```python
from build123d import *

# Parameters (mm, degrees)
SKETCH1_W           = 600
SKETCH1_H           = 540
BOSS_EXTRUDE1_DEPTH = 15
SKETCH2_W           = 175
SKETCH2_H           = 75.5
CUT_EXTRUDE1_DEPTH  = 404.887360535
SKETCH4_W           = 17
SKETCH4_H           = 32
CUT_EXTRUDE3_DEPTH  = 404.887360535
FILLET3_R           = 10
SKETCH5_W           = 40
SKETCH5_H           = 6
BOSS_EXTRUDE2_DEPTH = 15
SKETCH6_R           = 2.5
CUT_EXTRUDE4_DEPTH  = 404.887360535
BOSS_EXTRUDE3_DEPTH = 15
FILLET4_R           = 35
CUT_EXTRUDE5_DEPTH  = 15
FILLET5_R           = 7
SKETCH9_W           = 600
SKETCH9_H           = 5.5
CUT_EXTRUDE6_DEPTH  = 497.235831032
FILLET7_R           = 10
FILLET8_R           = 2
SKETCH10_W          = 90
SKETCH10_H          = 178
CUT_EXTRUDE7_DEPTH  = 15
FILLET9_R           = 5
SKETCH11_R          = 2.1
CUT_EXTRUDE8_DEPTH  = 15
SKETCH12_R          = 2
CUT_EXTRUDE9_DEPTH  = 497.235831032
SKETCH13_R          = 2
CUT_EXTRUDE10_DEPTH = 497.235831032


with BuildPart() as part:
    # Sketch1 → Boss-Extrude1 (new body)
    with BuildSketch(Plane.XY):
        Rectangle(SKETCH1_W, SKETCH1_H)
    extrude(amount=BOSS_EXTRUDE1_DEPTH)

    # Sketch2 → Cut-Extrude1 (cut, through all)
    with BuildSketch(Plane.XY.offset(15)):
        with Locations((-186, -232.25)):
            Rectangle(SKETCH2_W, SKETCH2_H)
        with Locations((186, -232.25)):
            Rectangle(SKETCH2_W, SKETCH2_H)
    extrude(amount=-CUT_EXTRUDE1_DEPTH, mode=Mode.SUBTRACT)

    # Sketch4 → Cut-Extrude3 (cut, through all)
    with BuildSketch(Plane.XY.offset(15)):
        with Locations((-259.5, 244.5)):
            Rectangle(SKETCH4_W, SKETCH4_H)
        with Locations((-112.5, 244.5)):
            Rectangle(SKETCH4_W, SKETCH4_H)
        with Locations((-259.5, -55.5)):
            Rectangle(SKETCH4_W, SKETCH4_H)
        with Locations((-112.5, -55.5)):
            Rectangle(SKETCH4_W, SKETCH4_H)
        with Locations((112.5, -55.5)):
            Rectangle(SKETCH4_W, SKETCH4_H)
        with Locations((259.5, -55.5)):
            Rectangle(SKETCH4_W, SKETCH4_H)
        with Locations((112.5, 244.5)):
            Rectangle(SKETCH4_W, SKETCH4_H)
        with Locations((259.5, 244.5)):
            Rectangle(SKETCH4_W, SKETCH4_H)
    extrude(amount=-CUT_EXTRUDE3_DEPTH, mode=Mode.SUBTRACT)

    # Fillet3
    fillet3_edges = [part.edges().sort_by_distance(p)[0] for p in [
        (-273.5, -194.5, 7.5),
        (-98.5, -194.5, 7.5),
        (98.5, -194.5, 7.5),
        (273.5, -194.5, 7.5),
    ]]
    fillet(fillet3_edges, radius=FILLET3_R)

    # Sketch5 → Boss-Extrude2 (add)
    with BuildSketch(Plane.XY.offset(15)):
        with Locations((-186, -197.5)):
            Rectangle(SKETCH5_W, SKETCH5_H)
        with Locations((186, -197.5)):
            Rectangle(SKETCH5_W, SKETCH5_H)
    extrude(amount=-BOSS_EXTRUDE2_DEPTH)

    # Sketch6 → Cut-Extrude4 (cut, through all)
    with BuildSketch(Plane.XY.offset(15)):
        with Locations((58.3, 117)):
            Circle(SKETCH6_R)
        with Locations((58.3, 103)):
            Circle(SKETCH6_R)
    extrude(amount=-CUT_EXTRUDE4_DEPTH, mode=Mode.SUBTRACT)

    # Sketch7 → Boss-Extrude3 (add)
    with BuildSketch(Plane.XY.offset(15)):
        Polygon((-300, 270), (300, 270), (175, 395), (-175, 395), align=None)
    extrude(amount=-BOSS_EXTRUDE3_DEPTH)

    # Fillet4
    fillet4_edges = [part.edges().sort_by_distance(p)[0] for p in [
        (-175, 395, 7.5),
        (175, 395, 7.5),
        (-300, 270, 7.5),
        (300, 270, 7.5),
    ]]
    fillet(fillet4_edges, radius=FILLET4_R)

    # Sketch8 → Cut-Extrude5 (cut)
    with BuildSketch(Plane.XY.offset(15)):
        Polygon((-230, 286.966991411), (-150, 286.966991411), (-150, 366.966991411), align=None)
        Polygon((150, 366.966991411), (230, 286.966991411), (150, 286.966991411), align=None)
    extrude(amount=-CUT_EXTRUDE5_DEPTH, mode=Mode.SUBTRACT)

    # Fillet5
    fillet5_edges = [part.edges().sort_by_distance(p)[0] for p in [
        (-230, 286.966991411, 7.5),
        (-150, 366.966991411, 7.5),
        (-150, 286.966991411, 7.5),
        (150, 286.966991411, 7.5),
        (150, 366.966991411, 7.5),
        (230, 286.966991411, 7.5),
    ]]
    fillet(fillet5_edges, radius=FILLET5_R)

    # Sketch9 → Cut-Extrude6 (cut, through all)
    with BuildSketch(Plane.XY.offset(15)):
        with Locations((0, -267.25)):
            Rectangle(SKETCH9_W, SKETCH9_H)
    extrude(amount=-CUT_EXTRUDE6_DEPTH, mode=Mode.SUBTRACT)

    # Fillet7
    fillet7_edges = [part.edges().sort_by_distance(p)[0] for p in [
        (-300, -264.5, 7.5),
        (300, -264.5, 7.5),
    ]]
    fillet(fillet7_edges, radius=FILLET7_R)

    # Fillet8
    fillet8_edges = [part.edges().sort_by_distance(p)[0] for p in [
        (-98.5, -264.5, 7.5),
        (98.5, -264.5, 7.5),
        (273.5, -264.5, 7.5),
        (-273.5, -264.5, 7.5),
    ]]
    fillet(fillet8_edges, radius=FILLET8_R)

    # Sketch10 → Cut-Extrude7 (cut)
    with BuildSketch(Plane.XY.offset(15)):
        with Locations((0, -135.5)):
            Rectangle(SKETCH10_W, SKETCH10_H)
    extrude(amount=-CUT_EXTRUDE7_DEPTH, mode=Mode.SUBTRACT)

    # Fillet9
    fillet9_edges = [part.edges().sort_by_distance(p)[0] for p in [
        (-45, -224.5, 7.5),
        (-45, -46.5, 7.5),
        (45, -46.5, 7.5),
        (45, -224.5, 7.5),
    ]]
    fillet(fillet9_edges, radius=FILLET9_R)

    # Sketch11 → Cut-Extrude8 (cut)
    with BuildSketch(Plane.XY.offset(15)):
        with Locations((53, -69.5)):
            Circle(SKETCH11_R)
        with Locations((53, -209.5)):
            Circle(SKETCH11_R)
        with Locations((-53, -209.5)):
            Circle(SKETCH11_R)
        with Locations((-53, -69.5)):
            Circle(SKETCH11_R)
    extrude(amount=-CUT_EXTRUDE8_DEPTH, mode=Mode.SUBTRACT)

    # Sketch12 → Cut-Extrude9 (cut, through all)
    with BuildSketch(Plane.XY.offset(15)):
        with Locations((-251.707106781, 259.792893219)):
            Circle(SKETCH12_R)
        with Locations((-267.292893219, 259.792893219)):
            Circle(SKETCH12_R)
        with Locations((-267.292893219, 229.207106781)):
            Circle(SKETCH12_R)
        with Locations((-251.707106781, 229.207106781)):
            Circle(SKETCH12_R)
        with Locations((-104.707106781, 259.792893219)):
            Circle(SKETCH12_R)
        with Locations((-120.292893219, 259.792893219)):
            Circle(SKETCH12_R)
        with Locations((-120.292893219, 229.207106781)):
            Circle(SKETCH12_R)
        with Locations((-104.707106781, 229.207106781)):
            Circle(SKETCH12_R)
        with Locations((-104.707106781, -40.207106781)):
            Circle(SKETCH12_R)
        with Locations((-120.292893219, -40.207106781)):
            Circle(SKETCH12_R)
        with Locations((-120.292893219, -70.792893219)):
            Circle(SKETCH12_R)
        with Locations((-104.707106781, -70.792893219)):
            Circle(SKETCH12_R)
        with Locations((-251.707106781, -40.207106781)):
            Circle(SKETCH12_R)
        with Locations((-267.292893219, -40.207106781)):
            Circle(SKETCH12_R)
        with Locations((-267.292893219, -70.792893219)):
            Circle(SKETCH12_R)
        with Locations((-251.707106781, -70.792893219)):
            Circle(SKETCH12_R)
        with Locations((251.707106781, -70.792893219)):
            Circle(SKETCH12_R)
        with Locations((267.292893219, -70.792893219)):
            Circle(SKETCH12_R)
        with Locations((267.292893219, -40.207106781)):
            Circle(SKETCH12_R)
        with Locations((251.707106781, -40.207106781)):
            Circle(SKETCH12_R)
        with Locations((104.707106781, -70.792893219)):
            Circle(SKETCH12_R)
        with Locations((120.292893219, -70.792893219)):
            Circle(SKETCH12_R)
        with Locations((120.292893219, -40.207106781)):
            Circle(SKETCH12_R)
        with Locations((104.707106781, -40.207106781)):
            Circle(SKETCH12_R)
        with Locations((104.707106781, 229.207106781)):
            Circle(SKETCH12_R)
        with Locations((120.292893219, 229.207106781)):
            Circle(SKETCH12_R)
        with Locations((120.292893219, 259.792893219)):
            Circle(SKETCH12_R)
        with Locations((104.707106781, 259.792893219)):
            Circle(SKETCH12_R)
        with Locations((251.707106781, 229.207106781)):
            Circle(SKETCH12_R)
        with Locations((267.292893219, 229.207106781)):
            Circle(SKETCH12_R)
        with Locations((267.292893219, 259.792893219)):
            Circle(SKETCH12_R)
        with Locations((251.707106781, 259.792893219)):
            Circle(SKETCH12_R)
    extrude(amount=-CUT_EXTRUDE9_DEPTH, mode=Mode.SUBTRACT)

    # Sketch13 → Cut-Extrude10 (cut, through all)
    with BuildSketch(Plane.XY.offset(15)):
        with Locations((-206.707106781, -195.207106781)):
            Circle(SKETCH13_R)
        with Locations((-165.292893219, -195.207106781)):
            Circle(SKETCH13_R)
        with Locations((165.292893219, -195.207106781)):
            Circle(SKETCH13_R)
        with Locations((206.707106781, -195.207106781)):
            Circle(SKETCH13_R)
    extrude(amount=-CUT_EXTRUDE10_DEPTH, mode=Mode.SUBTRACT)


solid = part.part
```
Part model, mm, in its own coordinate system. A direction names the side the tool comes from. Give positions to 0.01 mm unless a question says otherwise; leave off trailing zeros. Write each loop counter-clockwise with the first axis right and the second up, starting at its lowest first coordinate (ties: lowest second). Pieces come first, ordered by that corner, then holes. Notation, with made-up numbers: (-21, -8) -> (-11, -8) arc R31 ccw to (-11, 16) -> close; hole circle Ø9 at (58.25, 71.5). An arc over 180 degrees is marked (long way). Put each result on its own line as item: value. Start each with the question number.
Item 1: Cut at D-D (z = 5.25). State how many separate pieces and enclosed holes the cut face has, then the cut area to 3 significant figures.
Item 2: Cut at B-B (y = -167.5). List the corners of the cut face in (x, z), then the cut area to 3 significant figures.
Item 3: Cut at A-A (x = -5.5). List the corners of the cut face in (y, z).
Item 4: Which spindle directions (+Z, -Z, +X, -X, +Y, -Y) get a long thin tool onto all of the face, cutting with end or side? Do faces 1 (the face through (186, -200.5, 8)), 2 (the face through (189.607, 327.36, 7.605)), 3 (the face through (-4, 70, 15)). Say none if no direction does.
Item 5: Cut at C-C (y = 314.5). List the corners of the cut face in (x, z), then the cut area to 3 significant figures.
Item 6: Wall check: L1, parallel to Y at x = 58.3, z = 7.25; L2, parallel to X at y = -218.5, z = 4.75; L3, parallel to Y at x = 254, z = 1.25. Give the ranges that are in metal, low to high. Write a range as [from, to].
Item 7: Pull direction X, two halves, no side cores. Call faces 4 (the face through (-4, 70, 0)), 5 (the face through (-300, -3, 7)), 6 (the face through (104, -56, 8)): pulls with the +X half, pulls with the -X half, needs draft (parallel to the pull), parting line crosses it, or undercut.
Item 8: Pin check, flat tips, straight feed: pin 1 Ø6 at (x, z) = (-195, 7) entering from -Y; pin 2 Ø4.5 at (x, z) = (144.5, 9) entering from -Y; pin 3 Ø6 at (x, z) = (-110.5, 5.5) entering from -Y. Stop position of each tip, or through.
Answer list:
1. separate pieces: 1
1. enclosed holes: 17
1. area: 329,000 mm2
2. outline: (-300, 0) -> (-45, 0) -> (-45, 15) -> (-300, 15) -> close; (45, 0) -> (300, 0) -> (300, 15) -> (45, 15) -> close
2. area: 7,650 mm2
3. outline: (-264.5, 0) -> (-224.5, 0) -> (-224.5, 15) -> (-264.5, 15) -> close; (-46.5, 0) -> (395, 0) -> (395, 15) -> (-46.5, 15) -> close
4. face 1: +Z, -Z, -Y
4. face 2: +Z, -Z
4. face 3: +Z, +X, -X, +Y, -Y
5. outline: (-255.5, 0) -> (-202.47, 0) -> (-202.47, 15) -> (-255.5, 15) -> close; (-150, 0) -> (150, 0) -> (150, 15) -> (-150, 15) -> close; (202.47, 0) -> (255.5, 0) -> (255.5, 15) -> (202.47, 15) -> close
5. area: 6,090 mm2
6. L1: y = [-264.5, 100.5], [105.5, 114.5], [119.5, 395]
6. L2: x = [-300, -273.5], [-98.5, -45], [45, 98.5], [273.5, 300]
6. L3: y = [-194.5, -71.5], [-39.5, 228.5], [260.5, 316]
7. face 4: needs draft
7. face 5: pulls with the -X half
7. face 6: undercut
8. pin 1: stops at y = -200.5
8. pin 2: stops at y = -194.5
8. pin 3: stops at y = -194.55
